Verification items for the finished model (mm, model axes). Face numbers are marked on the shaded views. A direction names the side the tool comes from. Round coordinates to 2 decimals unless told otherwise and drop trailing zeros. Write each loop counter-clockwise with the first axis right and the second up, starting at its lowest first coordinate (ties: lowest second). Pieces come first, ordered by that corner, then holes. Notation, with made-up numbers: (36, 29.5) - (63, 29.5) arc R28 ccw to (63, 61.5) - close; hole circle Ø9 at (68, 15). An arc over 180 degrees is marked (long way). Answer as a JSON object with one key per item and string values.
```python
from build123d import *

# Parameters (mm, degrees)
SKETCH_4_W                = 46
SKETCH_4_H                = 107.5
EXTRUDE_1_DEPTH           = 3
SKETCH_5_W                = 23.5
SKETCH_5_H                = 63
EXTRUDE_2_DEPTH           = 12.4
SKETCH_6_R                = 1.75
CUT_EXTRUDE_1_DEPTH       = 66.1949768
SKETCH_6_3_R              = 3
CUT_EXTRUDE_2_DEPTH       = 2.7
CUT_EXTRUDE_START         = -20.8
SKETCH_6_4_R              = 3
CUT_EXTRUDE_3_DEPTH       = 2.7
SKETCH_6_5_R              = 3
CUT_EXTRUDE_4_DEPTH       = 2.7
SKETCH_6_6_R              = 3
CUT_EXTRUDE_5_DEPTH       = 2.7
SKETCH_7_R                = 0.7
CUT_EXTRUDE_6_DEPTH       = 2
CUT_EXTRUDE_START_2       = -2
SKETCH_8_W                = 16.4
SKETCH_8_H                = 14.4
CUT_EXTRUDE_7_DEPTH       = 59.458436136
SKETCH_9_W                = 46
SKETCH_9_H                = 8
EXTRUDE_3_DEPTH           = 10
SKETCH_9_3_W              = 3
SKETCH_9_3_H              = 91.5
EXTRUDE_4_DEPTH           = 3
SKETCH_10_R               = 0.6
CUT_EXTRUDE_8_DEPTH       = 2
SKETCH_11_W               = 26.4
SKETCH_11_H               = 14.4
CUT_EXTRUDE_9_DEPTH       = 5
SKETCH_12_R               = 0.5
CUT_EXTRUDE_10_DEPTH      = 2
CUT_EXTRUDE_11_DEPTH      = 61.458436136
CUT_EXTRUDE_12_DEPTH      = 90.164580972
CUT_EXTRUDE_12_DEPTH_BACK = 90.164580972
SKETCH_14_W               = 46
SKETCH_14_H               = 3
SKETCH_15_OUTSIDE_W       = 71.516
SKETCH_15_OUTSIDE_H       = 133.016
SKETCH_15_OUTSIDE_W_2     = 23.5
SKETCH_15_OUTSIDE_H_2     = 63
CUT_EXTRUDE_15_DEPTH      = 60.764726219
SKETCH_16_W               = 23.5
SKETCH_16_H               = 3
SKETCH_16_R               = 1
EXTRUDE_5_DEPTH           = 2
CUT_EXTRUDE_START_3       = -1
SKETCH_17_R               = 5.75
CUT_EXTRUDE_16_DEPTH      = 3.4
CUT_EXTRUDE_START_4       = 0.4
SKETCH_18_R               = 8.25
CUT_EXTRUDE_17_DEPTH      = 2
SKETCH_19_R               = 3.25
CUT_EXTRUDE_18_DEPTH      = 4
SKETCH_20_R               = 5.75
CUT_EXTRUDE_19_DEPTH      = 3.4
CUT_EXTRUDE_START_5       = -4.7
SKETCH_21_R               = 1
CUT_EXTRUDE_20_DEPTH      = 3
CUT_EXTRUDE_START_6       = -10.7
SKETCH_21_2_R             = 1
CUT_EXTRUDE_21_DEPTH      = 3


with BuildPart() as part:
    # 草图4 → 凸台-拉伸1 (new body)
    with BuildSketch(Plane(origin=(0, 0, 0), x_dir=(1, 0, 0), z_dir=(0, 1, 0))):
        Rectangle(SKETCH_4_W, SKETCH_4_H)
    extrude(amount=EXTRUDE_1_DEPTH)

    # 草图5 → 凸台-拉伸2 (add)
    with BuildSketch(Plane.XZ):
        Rectangle(SKETCH_5_W, SKETCH_5_H)
    extrude(amount=EXTRUDE_2_DEPTH)

    # 草图6 → 切除-拉伸1 (cut, through all)
    with BuildSketch(Plane.ZY.offset(11.75)):
        with Locations((0, -12.4)):
            Circle(SKETCH_6_R)
        with Locations((25, -12.4)):
            Circle(SKETCH_6_R)
        with Locations((-25, -12.4)):
            Circle(SKETCH_6_R)
    extrude(amount=-CUT_EXTRUDE_1_DEPTH, mode=Mode.SUBTRACT)

    # 草图6<3> → 切除-拉伸2 (cut)
    with BuildSketch(Plane.ZY.offset(11.75)):
        with Locations((0, -12.4)):
            Circle(SKETCH_6_3_R)
    extrude(amount=-CUT_EXTRUDE_2_DEPTH, mode=Mode.SUBTRACT)

    # 草图6<4> → 切除-拉伸3 (cut)
    with BuildSketch(Plane.ZY.offset(11.75).offset(CUT_EXTRUDE_START)):
        with Locations((0, -12.4)):
            Circle(SKETCH_6_4_R)
    extrude(amount=-CUT_EXTRUDE_3_DEPTH, mode=Mode.SUBTRACT)

    # 草图6<5> → 切除-拉伸4 (cut)
    with BuildSketch(Plane.ZY.offset(11.75)):
        with Locations((25, -12.4)):
            Circle(SKETCH_6_5_R)
        with Locations((-25, -12.4)):
            Circle(SKETCH_6_5_R)
    extrude(amount=-CUT_EXTRUDE_4_DEPTH, mode=Mode.SUBTRACT)

    # 草图6<6> → 切除-拉伸5 (cut)
    with BuildSketch(Plane.ZY.offset(11.75).offset(CUT_EXTRUDE_START)):
        with Locations((25, -12.4)):
            Circle(SKETCH_6_6_R)
        with Locations((-25, -12.4)):
            Circle(SKETCH_6_6_R)
    extrude(amount=-CUT_EXTRUDE_5_DEPTH, mode=Mode.SUBTRACT)

    # 草图7 → 切除-拉伸6 (cut)
    with BuildSketch(Plane(origin=(0, -12.4, 0), x_dir=(-1, 0, 0), z_dir=(0, -1, 0))):
        with Locations(Location((9.249949764, -20, 0), (0, 0, 90))):
            Circle(SKETCH_7_R)
        with Locations(Location((-9.249949764, -20, 0), (0, 0, 90))):
            Circle(SKETCH_7_R)
        with Locations(Location((-9.249949764, -6, 0), (0, 0, 90))):
            Circle(SKETCH_7_R)
        with Locations(Location((9.249949764, -6, 0), (0, 0, 90))):
            Circle(SKETCH_7_R)
        with Locations(Location((9.249949764, 6, 0), (0, 0, 90))):
            Circle(SKETCH_7_R)
        with Locations(Location((-9.249949764, 6, 0), (0, 0, 90))):
            Circle(SKETCH_7_R)
        with Locations(Location((-9.249949764, 20, 0), (0, 0, 90))):
            Circle(SKETCH_7_R)
        with Locations(Location((9.249949764, 20, 0), (0, 0, 90))):
            Circle(SKETCH_7_R)
    extrude(amount=-CUT_EXTRUDE_6_DEPTH, mode=Mode.SUBTRACT)

    # 草图8 → 切除-拉伸7 (cut, through all)
    with BuildSketch(Plane.XZ.offset(12.4).offset(CUT_EXTRUDE_START_2)):
        Rectangle(SKETCH_8_W, SKETCH_8_H)
    extrude(amount=-CUT_EXTRUDE_7_DEPTH, mode=Mode.SUBTRACT)

    # 草图9 → 凸台-拉伸3 (add)
    with BuildSketch(Plane.XZ):
        with Locations((0, 49.75)):
            Rectangle(SKETCH_9_W, SKETCH_9_H)
        with Locations((0, -49.75)):
            Rectangle(SKETCH_9_W, SKETCH_9_H)
    extrude(amount=EXTRUDE_3_DEPTH)

    # 草图9<3> → 凸台-拉伸4 (add)
    with BuildSketch(Plane.XZ):
        with Locations((-21.5, 0)):
            Rectangle(SKETCH_9_3_W, SKETCH_9_3_H)
        with Locations((21.5, 0)):
            Rectangle(SKETCH_9_3_W, SKETCH_9_3_H)
    extrude(amount=EXTRUDE_4_DEPTH)

    # 草图10 → 切除-拉伸8 (cut)
    with BuildSketch(Plane.XY.offset(53.75)):
        with Locations((-7.5, 0)):
            Circle(SKETCH_10_R)
        with Locations((7.5, 0)):
            Circle(SKETCH_10_R)
    extrude(amount=-CUT_EXTRUDE_8_DEPTH, mode=Mode.SUBTRACT)

    # 草图11 → 切除-拉伸9 (cut)
    with BuildSketch(Plane(origin=(0, 3, 0), x_dir=(1, 0, 0), z_dir=(0, 1, 0))):
        Rectangle(SKETCH_11_W, SKETCH_11_H)
    extrude(amount=-CUT_EXTRUDE_9_DEPTH, mode=Mode.SUBTRACT)

    # 草图12 → 切除-拉伸10 (cut)
    with BuildSketch(Plane(origin=(0, -2, 0), x_dir=(1, 0, 0), z_dir=(0, 1, 0))):
        with Locations(Location((-9.875, 0, 0), (0, 0, 270))):
            Circle(SKETCH_12_R)
        with Locations(Location((9.875, 0, 0), (0, 0, 270))):
            Circle(SKETCH_12_R)
    extrude(amount=-CUT_EXTRUDE_10_DEPTH, mode=Mode.SUBTRACT)

    # 草图13 → 切除-拉伸11 (cut, through all)
    with BuildSketch(Plane.XZ.offset(12.4)):
        Polygon((-8.75, 2.6), (-6.75, 2.6), (-6.75, 5.75), (-3.55, 5.75), (-3.55, -5.75), (-6.75, -5.75), (-6.75, -2.6), (-8.75, -2.6), align=None)
    extrude(amount=-CUT_EXTRUDE_11_DEPTH, mode=Mode.SUBTRACT)

    # 草图14 → 切除-拉伸12 (cut, two sides: drawn at the far end of the back side and taken through both)
    with BuildSketch(Plane.XY.offset(31.5).offset(-CUT_EXTRUDE_12_DEPTH_BACK)):
        with Locations((0, 1.5)):
            Rectangle(SKETCH_14_W, SKETCH_14_H)
    extrude(amount=CUT_EXTRUDE_12_DEPTH + CUT_EXTRUDE_12_DEPTH_BACK, mode=Mode.SUBTRACT)


with BuildPart() as cut_extrude_12_piece_1:
    # of the separate pieces the step leaves, piece 1, a body of its own (cut_extrude_12_pieces)
    add(part.part.solids().sort_by_distance((-11.75, 0, 31.5))[0])

    # 草图16 → 凸台-拉伸5 (add)
    # profile 1 of 2: a face of its own
    with BuildSketch(Plane(origin=(0, 0, 0), x_dir=(1, 0, 0), z_dir=(0, 1, 0))):
        with Locations((0, 33)):
            Rectangle(SKETCH_16_W, SKETCH_16_H)
        with Locations(Location((-7.5, 33, 0), (0, 0, 270))):
            Circle(SKETCH_16_R, mode=Mode.SUBTRACT)
        with Locations(Location((7.5, 33, 0), (0, 0, 270))):
            Circle(SKETCH_16_R, mode=Mode.SUBTRACT)
    # profile 2 of 2: a face of its own
    with BuildSketch(Plane(origin=(0, 0, 0), x_dir=(1, 0, 0), z_dir=(0, 1, 0))):
        with Locations((0, -33)):
            Rectangle(SKETCH_16_W, SKETCH_16_H)
        with Locations(Location((-7.5, -33, 0), (0, 0, 270))):
            Circle(SKETCH_16_R, mode=Mode.SUBTRACT)
        with Locations(Location((7.5, -33, 0), (0, 0, 270))):
            Circle(SKETCH_16_R, mode=Mode.SUBTRACT)
    extrude(amount=-EXTRUDE_5_DEPTH)

    # 草图17 → 切除-拉伸16 (cut)
    with BuildSketch(Plane(origin=(9.05, 0, 0), x_dir=(0, 0, -1), z_dir=(1, 0, 0)).offset(CUT_EXTRUDE_START_3)):
        with Locations((0, -12.4)):
            Circle(SKETCH_17_R)
    extrude(amount=-CUT_EXTRUDE_16_DEPTH, mode=Mode.SUBTRACT)

    # 草图18 → 切除-拉伸17 (cut)
    with BuildSketch(Plane(origin=(4.65, 0, 0), x_dir=(0, 0, -1), z_dir=(1, 0, 0)).offset(CUT_EXTRUDE_START_4)):
        with Locations((-12.5, -12.4)):
            Circle(SKETCH_18_R)
        with Locations((12.5, -12.4)):
            Circle(SKETCH_18_R)
    extrude(amount=CUT_EXTRUDE_17_DEPTH, mode=Mode.SUBTRACT)

    # 草图19 → 切除-拉伸18 (cut)
    with BuildSketch(Plane(origin=(5.05, 0, 0), x_dir=(0, 0, -1), z_dir=(1, 0, 0))):
        with Locations((-12.5, -12.4)):
            Circle(SKETCH_19_R)
        with Locations((12.5, -12.4)):
            Circle(SKETCH_19_R)
    extrude(amount=-CUT_EXTRUDE_18_DEPTH, mode=Mode.SUBTRACT)

    # 草图20 → 切除-拉伸19 (cut)
    with BuildSketch(Plane.ZY.offset(-7.05)):
        with Locations((-25, -12.4)):
            Circle(SKETCH_20_R)
        with Locations((25, -12.4)):
            Circle(SKETCH_20_R)
    extrude(amount=CUT_EXTRUDE_19_DEPTH, mode=Mode.SUBTRACT)

    # 草图21 → 切除-拉伸20 (cut)
    with BuildSketch(Plane(origin=(11.75, 0, 0), x_dir=(0, 0, -1), z_dir=(1, 0, 0)).offset(CUT_EXTRUDE_START_5)):
        with Locations((-12.5, -12.4)):
            Circle(SKETCH_21_R)
        with Locations((12.5, -12.4)):
            Circle(SKETCH_21_R)
    extrude(amount=CUT_EXTRUDE_20_DEPTH, mode=Mode.SUBTRACT)

    # 草图21<2> → 切除-拉伸21 (cut)
    with BuildSketch(Plane(origin=(11.75, 0, 0), x_dir=(0, 0, -1), z_dir=(1, 0, 0)).offset(CUT_EXTRUDE_START_6)):
        with Locations((-12.5, -12.4)):
            Circle(SKETCH_21_2_R)
        with Locations((12.5, -12.4)):
            Circle(SKETCH_21_2_R)
    extrude(amount=-CUT_EXTRUDE_21_DEPTH, mode=Mode.SUBTRACT)


with BuildPart() as cut_extrude_12_piece_2:
    # of the separate pieces the step leaves, piece 2, a body of its own (cut_extrude_12_pieces)
    add(part.part.solids().sort_by_distance((-23, 0, 53.75))[0])

    # 草图15 outside → 切除-拉伸15 (cut, through all)
    with BuildSketch(Plane.XZ.offset(12.4)):
        Rectangle(SKETCH_15_OUTSIDE_W, SKETCH_15_OUTSIDE_H)
        Rectangle(SKETCH_15_OUTSIDE_W_2, SKETCH_15_OUTSIDE_H_2, mode=Mode.SUBTRACT)
    extrude(amount=-CUT_EXTRUDE_15_DEPTH, mode=Mode.SUBTRACT)


solid = cut_extrude_12_piece_1.part
```
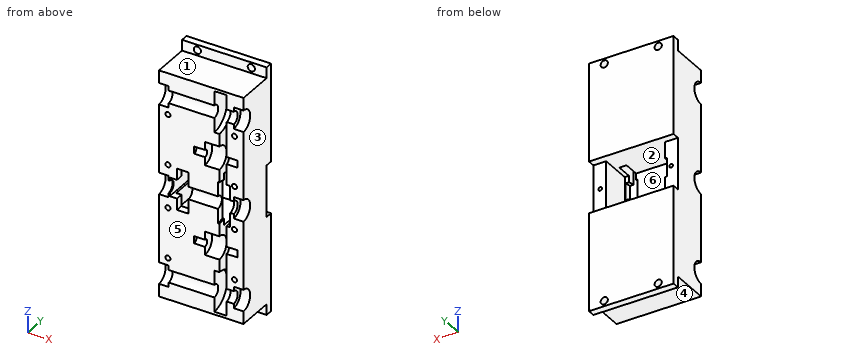
Q1. Set-up check for the marked faces 1, 2 and 3: record each of +Z, -Z, +X, -X, +Y, -Y from which the full face is reachable in a straight line by a thin tool's end or side.
Geometry check:
{"face 1": "+Z, +X, -X, -Y", "face 2": "+Y", "face 3": "+Z, -Z, +X, +Y, -Y"}
Q2. Release check for a two-part mould opening along Z. For the marked faces 4, 5 and 6 record: released by +Z, released by -Z, zero draft, split by the parting line, or undercut.
Geometry check:
{"face 4": "released by -Z", "face 5": "zero draft", "face 6": "undercut"}
Q3. Section check D-D, the plane x = -0.5. Record the cut outline in (y, z).
Geometry check:
{"outline": "(-12.4, -31.5) - (-2, -31.5) - (-2, -34.5) - (0, -34.5) - (0, -7.2) - (-10.4, -7.2) - (-10.4, 7.2) - (0, 7.2) - (0, 34.5) - (-2, 34.5) - (-2, 31.5) - (-12.4, 31.5) - (-12.4, 26.75) arc R1.75 cw to (-12.4, 23.25) - (-12.4, 13.5) arc R1 cw to (-12.4, 11.5) - (-12.4, 1.75) arc R1.75 cw to (-12.4, -1.75) - (-12.4, -11.5) arc R1 cw to (-12.4, -13.5) - (-12.4, -23.25) arc R1.75 cw to (-12.4, -26.75) - close"}
Q4. Section check A-A, the plane x = 3. Record the cut outline in (y, z), then the cut area to 3 significant figures.
Geometry check:
{"outline": "(-12.4, -31.5) - (-2, -31.5) - (-2, -34.5) - (0, -34.5) - (0, -7.2) - (-10.4, -7.2) - (-10.4, 7.2) - (0, 7.2) - (0, 34.5) - (-2, 34.5) - (-2, 31.5) - (-12.4, 31.5) - (-12.4, 26.75) arc R1.75 cw to (-12.4, 23.25) - (-12.4, 15.75) arc R3.25 cw to (-12.4, 9.25) - (-12.4, 1.75) arc R1.75 cw to (-12.4, -1.75) - (-12.4, -9.25) arc R3.25 cw to (-12.4, -15.75) - (-12.4, -23.25) arc R1.75 cw to (-12.4, -26.75) - close", "area": "596 mm2"}
Q5. Section check B-B, the plane z = 12.5. Record the cut outline in (x, y), then the cut area to 3 significant figures.
Geometry check:
{"outline": "(-11.75, -12.4) - (-1.95, -12.4) - (-1.95, -11.4) - (1.05, -11.4) - (1.05, -9.15) - (5.05, -9.15) - (5.05, -4.15) - (7.05, -4.15) - (7.05, -11.4) - (10.05, -11.4) - (10.05, -12.4) - (11.75, -12.4) - (11.75, 0) - (-11.75, 0) - close", "area": "256 mm2"}
Q6. Section check C-C, the plane y = -7.25. Record the cut outline in (x, z), then the cut area to 3 significant figures.
Geometry check:
{"outline": "(-11.75, -31.5) - (11.75, -31.5) - (11.75, 31.5) - (-11.75, 31.5) - close; hole (-8.75, -2.6) - (-8.2, -2.6) - (-8.2, -7.2) - (5.05, -7.2) - (5.05, -18.95) - (7.05, -18.95) - (7.05, -7.2) - (8.2, -7.2) - (8.2, 7.2) - (7.05, 7.2) - (7.05, 18.95) - (5.05, 18.95) - (5.05, 7.2) - (-8.2, 7.2) - (-8.2, 2.6) - (-8.75, 2.6) - close; hole (3.65, -27.56) - (7.05, -27.56) - (7.05, -22.44) - (3.65, -22.44) - close; hole (3.65, 22.44) - (7.05, 22.44) - (7.05, 27.56) - (3.65, 27.56) - close", "area": "1,160 mm2"}
Q7. Gauge pin test, flat ends, axial feed: P1, Ø2, axis at x = 9, z = 18.5, coming from the +Y side; P2, Ø10.5, axis at x = 0, z = -0.5, coming from the +Y side; P3, Ø2.5, axis at x = 7.5, z = 33, coming from the -Y side; P4, Ø1.6, axis at y = -11.5, z = 1, coming from the -X side. Record the tip position at first contact, or that the pin passes through.
Geometry check:
{"P1": "stops at y = 0", "P2": "stops at y = -10.4", "P3": "stops at y = -2", "P4": "stops at x = -9.05"}
Q8. Material ranges on line 1 along X through (y, z) = (-11.2, -6); line 2 along X through (y, z) = (-1.4, 33); line 3 along X through (y, z) = (-3.1, 0) (3 decimals), recorded low to high. Write a range as [from, to].
Geometry check:
{"line 1": "x = [-11.75, -9.95], [-8.55, 5.05], [7.05, 8.55], [9.95, 11.75]", "line 2": "x = [-11.75, -8.5], [-6.5, 6.5], [8.5, 11.75]", "line 3": "x = [-11.75, -10.375], [-9.375, -8.75], [8.2, 9.375], [10.375, 11.75]"}
